For this review, take the finished solid that the model builds, in its own axes (mm). A direction names the side the tool comes from. Coordinates: 2 decimals unless noted, no trailing zeros. Loops run counter-clockwise (first coordinate to the right, second up) from the corner with the lowest first, then second, coordinate; pieces in that order, holes last. Notation, with made-up numbers: (21, -14) - (60, -14) arc R28 cw to (60, 11) - close; hole circle Ø6 at (55, 87). An arc over 180 degrees is marked (long way). One line per item, written item: value. Start each with the question number.
1. Take a section at B-B, the plane z = 6. State the section outline as (x, y) points.
2. For faces 1 (the face through (0, 3, -48)), 2 (the face through (-1, 0, -1)), list the 3-axis set-ups (+Z, -Z, +X, -X, +Y, -Y) from which the entire face can be reached by the end or side of a thin tool; tool diameter is ignored.
3. Take a section at A-A, the plane x = -46.5. State the section outline as (y, z) points.
4. To check wall thickness, follow line 1 (X direction, y = 3.2, z = -4); line 2 (Z direction, x = -56, y = 3.7); line 3 (Y direction, x = -82.5, z = 26.5). State the ranges of each line that lie inside material, in increasing order. Write a range as from..to.
```python
from build123d import *

# Parameters (mm, degrees)
SKETCH_1_W      = 183
SKETCH_1_H      = 100
EXTRUDE_1_DEPTH = 3
SKETCH_2_W      = 165
SKETCH_2_H      = 89
EXTRUDE_2_DEPTH = 1
FILLET_1_R      = 10
FILLET_2_R      = 1.5
FILLET_3_R      = 0.2


with BuildPart() as part:
    # 草图1 → 凸台-拉伸1 (new body)
    with BuildSketch(Plane(origin=(0, 0, 0), x_dir=(1, 0, 0), z_dir=(0, 1, 0))):
        Rectangle(SKETCH_1_W, SKETCH_1_H)
    extrude(amount=EXTRUDE_1_DEPTH)

    # 草图2 → 凸台-拉伸2 (add)
    with BuildSketch(Plane(origin=(0, 3, 0), x_dir=(1, 0, 0), z_dir=(0, 1, 0))):
        Rectangle(SKETCH_2_W, SKETCH_2_H)
    extrude(amount=EXTRUDE_2_DEPTH)

    # 圆角1
    fillet_1_edges = [part.edges().sort_by_distance(p)[0] for p in [
        (-82.5, 3.5, -44.5),
        (-82.5, 3.5, 44.5),
        (82.5, 3.5, 44.5),
        (82.5, 3.5, -44.5),
    ]]
    fillet(fillet_1_edges, radius=FILLET_1_R)

    # 圆角2
    # the kernel refuses this fillet: 1.5 mm, written as the material it adds along each edge
    with BuildSketch(Plane(origin=(-72.5, 3, 34.5), x_dir=(-1, 0, 0), z_dir=(0, 0, -1))) as fillet_2_piece_1:
        with BuildLine():
            CenterArc((11.414213562, 1.5), FILLET_2_R, 199.471220634, 70.528779366)
            Line((10, 1), (9.971715729, 0.99))
            ThreePointArc((9.971715729, 0.99), (9.97, 0.5), (9.97, 0))
            Line((9.97, 0), (10, -0.03))
            Line((10, -0.03), (11.414213562, -0.03))
            Line((11.414213562, -0.03), (11.414213562, 0))
        make_face()
    revolve(axis=Axis((-72.5, 3, 34.5), (0, 1, 0)), revolution_arc=90)
    with BuildSketch(Plane(origin=(-82.5, 3, -34.5), x_dir=(-1, 0, 0), z_dir=(0, 0, 1)), Plane(origin=(82.5, 3, 34.5), x_dir=(1, 0, 0), z_dir=(0, 0, -1))) as fillet_2_piece_2:
        with BuildLine():
            CenterArc((1.414213562, -1.5), FILLET_2_R, 90, 70.528779366)
            Line((0, -1), (-0.028284271, -0.99))
            ThreePointArc((-0.028284271, -0.99), (-0.03, -0.5), (-0.03, 0))
            Line((-0.03, 0), (0, 0.03))
            Line((0, 0.03), (1.414213562, 0.03))
            Line((1.414213562, 0.03), (1.414213562, 0))
        make_face()
    extrude(amount=69)
    with BuildSketch(Plane(origin=(-72.5, 3, -34.5), x_dir=(0, 0, -1), z_dir=(1, 0, 0))) as fillet_2_piece_3:
        with BuildLine():
            CenterArc((11.414213562, 1.5), FILLET_2_R, 199.471220634, 70.528779366)
            Line((10, 1), (9.971715729, 0.99))
            ThreePointArc((9.971715729, 0.99), (9.97, 0.5), (9.97, 0))
            Line((9.97, 0), (10, -0.03))
            Line((10, -0.03), (11.414213562, -0.03))
            Line((11.414213562, -0.03), (11.414213562, 0))
        make_face()
    revolve(axis=Axis((-72.5, 3, -34.5), (0, 1, 0)), revolution_arc=90)
    with BuildSketch(Plane(origin=(72.5, 3, -44.5), x_dir=(0, 0, -1), z_dir=(-1, 0, 0)), Plane(origin=(-72.5, 3, 44.5), x_dir=(0, 0, 1), z_dir=(1, 0, 0))) as fillet_2_piece_4:
        with BuildLine():
            CenterArc((1.414213562, -1.5), FILLET_2_R, 90, 70.528779366)
            Line((0, -1), (-0.028284271, -0.99))
            ThreePointArc((-0.028284271, -0.99), (-0.03, -0.5), (-0.03, 0))
            Line((-0.03, 0), (0, 0.03))
            Line((0, 0.03), (1.414213562, 0.03))
            Line((1.414213562, 0.03), (1.414213562, 0))
        make_face()
    extrude(amount=145)
    with BuildSketch(Plane(origin=(72.5, 3, -34.5), x_dir=(0, 0, -1), z_dir=(-1, 0, 0))) as fillet_2_piece_5:
        with BuildLine():
            CenterArc((11.414213562, -1.5), FILLET_2_R, 90, 70.528779366)
            Line((10, -1), (9.971715729, -0.99))
            ThreePointArc((9.971715729, -0.99), (9.97, -0.5), (9.97, 0))
            Line((9.97, 0), (10, 0.03))
            Line((10, 0.03), (11.414213562, 0.03))
            Line((11.414213562, 0.03), (11.414213562, 0))
        make_face()
    revolve(axis=Axis((72.5, 3, -34.5), (0, -1, 0)), revolution_arc=90)
    with BuildSketch(Plane(origin=(72.5, 3, 34.5), x_dir=(0, 0, 1), z_dir=(-1, 0, 0))) as fillet_2_piece_6:
        with BuildLine():
            CenterArc((11.414213562, 1.5), FILLET_2_R, 199.471220634, 70.528779366)
            Line((10, 1), (9.971715729, 0.99))
            ThreePointArc((9.971715729, 0.99), (9.97, 0.5), (9.97, 0))
            Line((9.97, 0), (10, -0.03))
            Line((10, -0.03), (11.414213562, -0.03))
            Line((11.414213562, -0.03), (11.414213562, 0))
        make_face()
    revolve(axis=Axis((72.5, 3, 34.5), (0, 1, 0)), revolution_arc=90)

    # 圆角3
    fillet_3_edges = [part.edges().sort_by_distance(p)[0] for p in [
        (-82.5, 4, 0),
        (0, 4, -44.5),
        (0, 4, 44.5),
        (82.5, 4, 0),
        (-79.571067812, 4, 41.571067812),
        (79.571067812, 4, 41.571067812),
        (79.571067812, 4, -41.571067812),
        (-79.571067812, 4, -41.571067812),
    ]]
    fillet(fillet_3_edges, radius=FILLET_3_R)


solid = part.part
```
Solutions:
1. outline: (-91.5, 0) - (91.5, 0) - (91.5, 3) - (83.91, 3) arc R1.5 cw to (82.55, 3.88) arc R0.2 ccw to (82.37, 4) - (-82.37, 4) arc R0.2 ccw to (-82.55, 3.88) arc R1.5 cw to (-83.91, 3) - (-91.5, 3) - close
2. face 1: +Y
2. face 2: +Z, -Z, +X, -X, -Y
3. outline: (0, -50) - (3, -50) - (3, -45.91) arc R1.5 cw to (3.88, -44.55) arc R0.2 ccw to (4, -44.37) - (4, 44.37) arc R0.2 ccw to (3.88, 44.55) arc R1.5 cw to (3, 45.91) - (3, 50) - (0, 50) - close
4. line 1: -83.17..83.17
4. line 2: -44.65..44.65
4. line 3: 0..3.95
